from build123d import *

# Parameters (mm, degrees)
SKETCH_W        = 136
SKETCH_H        = 44
PAD_DEPTH       = 3
SKETCH001_W     = 14
SKETCH001_H     = 12.5
SKETCH001_W_2   = 56
SKETCH001_H_2   = 11
SKETCH001_W_3   = 11.2
SKETCH001_H_3   = 13
POCKET_DEPTH    = 3.001
SKETCH002_R     = 1.25
POCKET001_DEPTH = 3.001
FILLET_R        = 2


with BuildPart() as part:
    # Sketch → Pad (new body)
    with BuildSketch(Plane.XZ):
        with Locations((68, 22)):
            Rectangle(SKETCH_W, SKETCH_H)
    extrude(amount=PAD_DEPTH)

    # Sketch001 (on Face6 of Pad) → Pocket (cut, through all)
    with BuildSketch(Plane.XZ.offset(3)):
        with Locations((56.56, 12.25)):
            Rectangle(SKETCH001_W, SKETCH001_H)
        with Locations((75, 25.5)):
            Rectangle(SKETCH001_W_2, SKETCH001_H_2)
        with Locations((86.5, 12.5)):
            Rectangle(SKETCH001_W_3, SKETCH001_H_3)
    extrude(amount=-POCKET_DEPTH, mode=Mode.SUBTRACT)

    # Sketch002 (on Face5 of Pocket) → Pocket001 (cut, through all)
    with BuildSketch(Plane.XZ.offset(3)):
        with Locations((5, 22)):
            Circle(SKETCH002_R)
        with Locations((131, 22)):
            Circle(SKETCH002_R)
    extrude(amount=-POCKET001_DEPTH, mode=Mode.SUBTRACT)

    # Fillet
    fillet_edges = [part.edges().sort_by_distance(p)[0] for p in [
        (47, -1.5, 31),
        (47, -1.5, 20),
        (103, -1.5, 20),
        (103, -1.5, 31),
        (92.1, -1.5, 19),
        (80.9, -1.5, 19),
        (80.9, -1.5, 6),
        (92.1, -1.5, 6),
        (63.56, -1.5, 6),
        (49.56, -1.5, 6),
        (49.56, -1.5, 18.5),
        (63.56, -1.5, 18.5),
    ]]
    fillet(fillet_edges, radius=FILLET_R)


solid = part.part
Can you work these out from the model? Positions are in its coordinate system, mm. A direction names the side the tool comes from. Round coordinates to 2 decimals unless told otherwise and drop trailing zeros. Write each loop counter-clockwise with the first axis right and the second up, starting at its lowest first coordinate (ties: lowest second). Pieces come first, ordered by that corner, then holes. Notation, with made-up numbers: M 75,83 L 104,83 A14 cw 104,108 Z; hole C 53,69 d9. An arc over 180 degrees is marked long. Use CSV: the item, a comma, the result in double quotes.
(1) We'd pull the mould along Z, two halves only. Please class faces 1 (the flat face through (75, -2, 31)), 2 (the flat face through (67, 0, 17)), 3 (the flat face through (67, -1, 0)): +Z half, -Z half, draft (parallel to the pull), parting line (faces both ways), or undercut.
Check values:
face 1,"undercut"
face 2,"draft"
face 3,"-Z half"
(2) I need wall thicknesses on line 1 along X through (y, z) = (-0.2, 16.5); line 2 along X through (y, z) = (-2, 27); line 3 along Z through (x, y) = (79, -2). Which ranges of each line are inside material? Lowest first, please.
Check values:
line 1,"0 to 49.56, 63.56 to 80.9, 92.1 to 136"
line 2,"0 to 47, 103 to 136"
line 3,"0 to 20, 31 to 44"
(3) Imagine slicing it at B-B (z = 15). Write out the boundary of the cut face in (x, y), plus the area to 3 significant figures.
Check values:
outline,"M 0,-3 L 49.56,-3 L 49.56,0 L 0,0 Z; M 63.56,-3 L 80.9,-3 L 80.9,0 L 63.56,0 Z; M 92.1,-3 L 136,-3 L 136,0 L 92.1,0 Z"
area,"332 mm^2"
(4) Imagine slicing it at A-A (x = 5). Write out the boundary of the cut face in (y, z), plus the area to 4 significant figures.
Check values:
outline,"M -3,0 L 0,0 L 0,20.75 L -3,20.75 Z; M -3,23.25 L 0,23.25 L 0,44 L -3,44 Z"
area,"124.5 mm^2"
(5) Imagine slicing it at C-C (y = -1.9). Count the separate pieces of the cut face and the enclosed holes in it, plus the area to 3 significant figures.
Check values:
separate pieces,"1"
enclosed holes,"5"
area,"5,050 mm^2"
(6) Imagine slicing it at D-D (x = 86.5). Write out the boundary of the cut face in (y, z).
Check values:
outline,"M -3,0 L 0,0 L 0,6 L -3,6 Z; M -3,19 L 0,19 L 0,20 L -3,20 Z; M -3,31 L 0,31 L 0,44 L -3,44 Z"
(7) On a 3-axis mill with a long thin cutter (end or side, diameter ignored), from which of +Z, -Z, +X, -X, +Y, -Y can I reach the whole of each face in a straight line? I mean faces 4 (the flat face through (0, -1, 22)), 5 (the flat face through (86, -2, 19)). Say none if no direction works.
Check values:
face 4,"+Z, -Z, -X, +Y, -Y"
face 5,"+Y, -Y"
